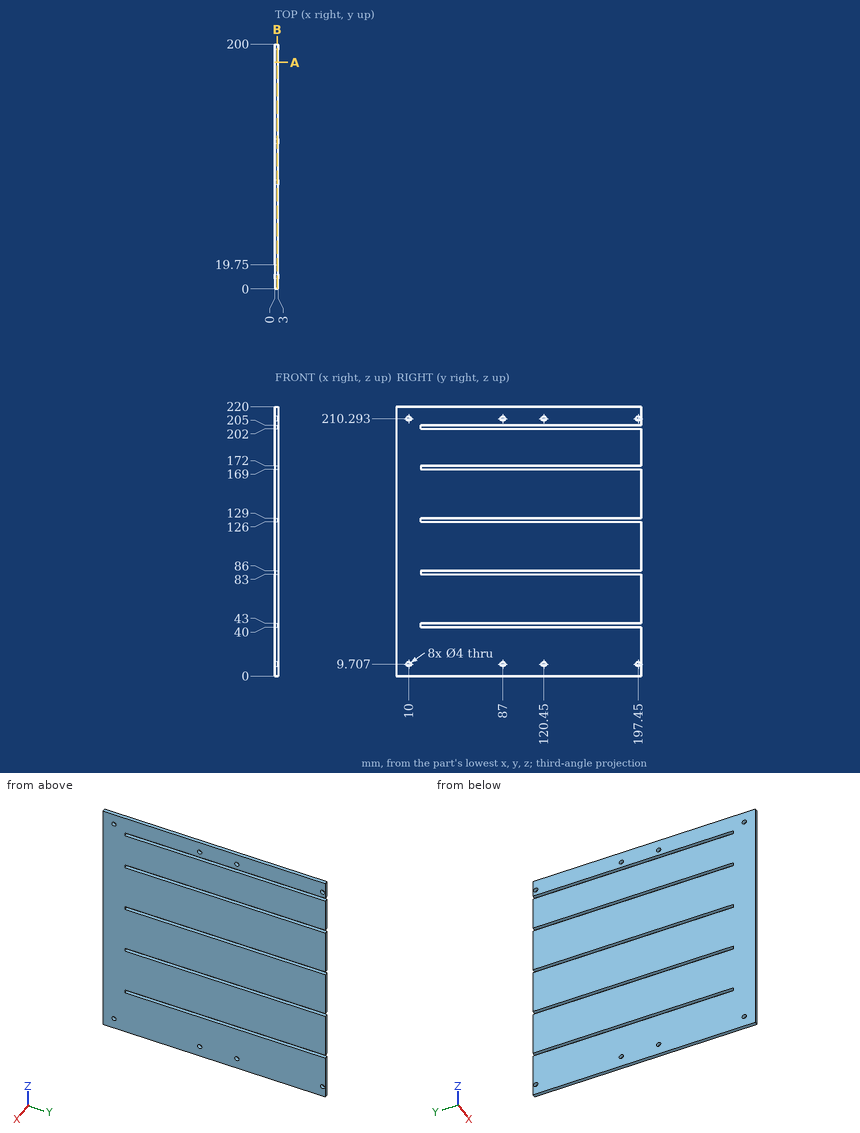
Print and shaded views of the part. All mm, measured from the part's lowest x, y and z. Give positions to 0.01 mm unless a question says otherwise; leave off trailing zeros. Order: outer loops, then holes, each group sorted by start corner. A loop starts at its lowest first (then second) coordinate and runs counter-clockwise, first axis right, second up. Notation, with made-up numbers: M -5.5,50 L 50.5,50 A8 cw 50.5,64 Z; hole C 0,64 d5. An arc over 180 degrees is marked long. Use one line per item in the form item = value.
Q1. Slice it at B-B, the plane x = 1.9. State how many separate pieces and enclosed holes the cut face has, and give its area (3 significant figures).
Conclusion:
separate_pieces = 1
enclosed_holes = 8
area = 41,200 mm2
Q2. Wall check: probe 1 along Z at (x, y) = (2.7, 25); probe 2 along Z at (x, y) = (1.6, 10); probe 3 along Y at (x, z) = (1.35, 41.5). Give the ranges that are in metal, low to high.
Conclusion:
probe_1 = 0 to 40, 43 to 83, 86 to 126, 129 to 169, 172 to 202, 205 to 220
probe_2 = 0 to 7.71, 11.71 to 208.29, 212.29 to 220
probe_3 = 0 to 19.75
Q3. Slice it at A-A, the plane y = 185. Write the cut outline in (x, z), and give its area (3 significant figures).
Conclusion:
outline = M 0,0 L 3,0 L 3,40 L 0,40 Z; M 0,43 L 3,43 L 3,83 L 0,83 Z; M 0,86 L 3,86 L 3,126 L 0,126 Z; M 0,129 L 3,129 L 3,169 L 0,169 Z; M 0,172 L 3,172 L 3,202 L 0,202 Z; M 0,205 L 3,205 L 3,220 L 0,220 Z
area = 615 mm2
Q4. Pin check, flat tips, straight feed: P1, Ø1, axis at y = 108.5, z = 197, coming from the -X side; P2, Ø1.5, axis at x = 1, z = 42, coming from the +Y side. Stop position of each tip, or through.
Conclusion:
P1 = 0
P2 = 19.75
